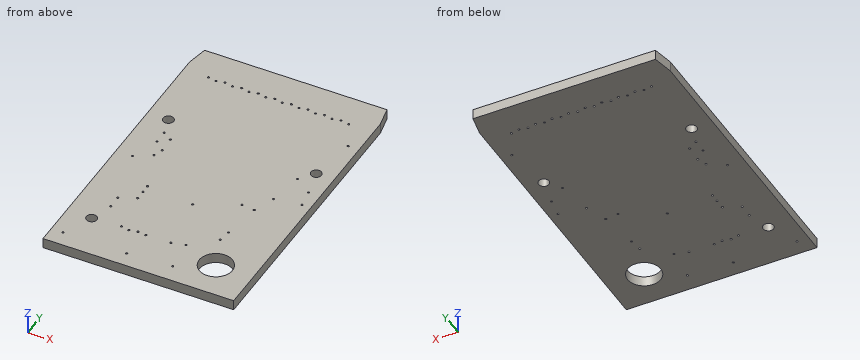
```python
from build123d import *

# Parameters (mm, degrees)
BOARD_OUTLINE_DEPTH = 0.7874
SKETCH2_R           = 0.0762
NPTH_DEPTH          = 1.7874
SKETCH3_R           = 0.405
SKETCH3_R_2         = 1.27
PTH_DEPTH           = 1.7874


with BuildPart() as part:
    # Sketch1 → Board_Outline (new body)
    with BuildSketch(Plane.XY):
        Polygon((14.605, 0), (0, 0), (0, 21.59), (0.3175, 23.1775), (14.2875, 23.1775), (14.605, 21.59), align=None)
    extrude(amount=BOARD_OUTLINE_DEPTH)

    # Sketch2 → NPTH (cut, through all)
    with BuildSketch(Plane.XY):
        with Locations((2.4638, 6.2738)):
            Circle(SKETCH2_R)
        with Locations((7.9248, 3.6068)):
            Circle(SKETCH2_R)
        with Locations((11.303, 9.3726)):
            Circle(SKETCH2_R)
        with Locations((10.3124, 9.4742)):
            Circle(SKETCH2_R)
        with Locations((13.7668, 18.4658)):
            Circle(SKETCH2_R)
        with Locations((1.27, 10.7442)):
            Circle(SKETCH2_R)
        with Locations((1.905, 20.701)):
            Circle(SKETCH2_R)
        with Locations((2.5146, 11.5062)):
            Circle(SKETCH2_R)
        with Locations((11.9126, 11.0236)):
            Circle(SKETCH2_R)
        with Locations((11.43, 20.574)):
            Circle(SKETCH2_R)
        with Locations((10.795, 20.701)):
            Circle(SKETCH2_R)
        with Locations((4.1148, 3.6322)):
            Circle(SKETCH2_R)
        with Locations((8.9408, 3.8608)):
            Circle(SKETCH2_R)
        with Locations((3.683, 8.3058)):
            Circle(SKETCH2_R)
        with Locations((4.7498, 3.5052)):
            Circle(SKETCH2_R)
        with Locations((12.065, 20.701)):
            Circle(SKETCH2_R)
        with Locations((10.16, 20.574)):
            Circle(SKETCH2_R)
        with Locations((9.525, 20.701)):
            Circle(SKETCH2_R)
        with Locations((8.89, 20.574)):
            Circle(SKETCH2_R)
        with Locations((10.7442, 5.4356)):
            Circle(SKETCH2_R)
        with Locations((3.683, 7.62)):
            Circle(SKETCH2_R)
        with Locations((9.1948, 1.397)):
            Circle(SKETCH2_R)
        with Locations((3.683, 6.858)):
            Circle(SKETCH2_R)
        with Locations((7.3152, 7.9756)):
            Circle(SKETCH2_R)
        with Locations((6.0198, 3.556)):
            Circle(SKETCH2_R)
        with Locations((5.3848, 3.6322)):
            Circle(SKETCH2_R)
        with Locations((8.255, 20.701)):
            Circle(SKETCH2_R)
        with Locations((7.62, 20.574)):
            Circle(SKETCH2_R)
        with Locations((6.985, 20.701)):
            Circle(SKETCH2_R)
        with Locations((6.35, 20.574)):
            Circle(SKETCH2_R)
        with Locations((5.715, 20.701)):
            Circle(SKETCH2_R)
        with Locations((5.08, 20.574)):
            Circle(SKETCH2_R)
        with Locations((4.445, 20.701)):
            Circle(SKETCH2_R)
        with Locations((3.81, 20.574)):
            Circle(SKETCH2_R)
        with Locations((3.175, 20.701)):
            Circle(SKETCH2_R)
        with Locations((2.54, 20.574)):
            Circle(SKETCH2_R)
        with Locations((2.0066, 13.97)):
            Circle(SKETCH2_R)
        with Locations((12.7, 20.574)):
            Circle(SKETCH2_R)
        with Locations((0.889, 1.2192)):
            Circle(SKETCH2_R)
        with Locations((13.6906, 12.7508)):
            Circle(SKETCH2_R)
        with Locations((2.0066, 12.9032)):
            Circle(SKETCH2_R)
        with Locations((12.3698, 13.716)):
            Circle(SKETCH2_R)
        with Locations((5.7912, 1.1938)):
            Circle(SKETCH2_R)
        with Locations((2.4638, 5.2324)):
            Circle(SKETCH2_R)
        with Locations((2.7178, 13.5128)):
            Circle(SKETCH2_R)
        with Locations((10.8712, 6.4008)):
            Circle(SKETCH2_R)
        with Locations((13.9192, 11.3538)):
            Circle(SKETCH2_R)
        with Locations((2.7686, 12.2428)):
            Circle(SKETCH2_R)
    extrude(amount=NPTH_DEPTH, mode=Mode.SUBTRACT)

    # Sketch3 → PTH (cut, through all)
    with BuildSketch(Plane.XY):
        with Locations((1.61, 15.37)):
            Circle(SKETCH3_R)
        with Locations((11.75, 2.86)):
            Circle(SKETCH3_R_2)
        with Locations((13.22, 14.81)):
            Circle(SKETCH3_R)
        with Locations((1.91, 3.49)):
            Circle(SKETCH3_R)
    extrude(amount=PTH_DEPTH, mode=Mode.SUBTRACT)


solid = part.part
```
Here's how the part is built. I have some questions about the finished solid (model axes, mm). Coordinates: 2 decimals unless noted, no trailing zeros. Loops run counter-clockwise (first coordinate to the right, second up) from the corner with the lowest first, then second, coordinate; pieces in that order, holes last. Notation, with made-up numbers: M -19,86.5 L 33,86.5 A21 cw 33,90.5 Z; hole C 44.25,0.25 d5. An arc over 180 degrees is marked long. One line per item, written item: value.
1. Please list where these lines run through material, in increasing order: probe 1 along Y at (x, z) = (12.7, 0.35); probe 2 along Y at (x, z) = (13.22, 0.3) (1 decimal); probe 3 along X at (y, z) = (14.81, 0.2) (3 decimals).
Geometry says:
probe 1: y = 0 to 2.02, 3.7 to 20.5, 20.65 to 23.18
probe 2: y = 0 to 14.4, 15.2 to 23.2
probe 3: x = 0 to 12.815, 13.625 to 14.605
2. Imagine slicing it at B-B (z = 0.5). State how many separate pieces and enclosed holes the cut face has, and give its area (3 significant figures).
Geometry says:
separate pieces: 1
enclosed holes: 52
area: 331 mm2
3. Imagine slicing it at A-A (y = 2.86). List the corners of the cut face in (x, z) for me (3 decimals), and give its area (3 significant figures).
Geometry says:
outline: M 0,0 L 10.48,0 L 10.48,0.787 L 0,0.787 Z; M 13.02,0 L 14.605,0 L 14.605,0.787 L 13.02,0.787 Z
area: 9.50 mm2
